```python
from build123d import *

# Parameters (mm, degrees)
EXTRUDE_1_DEPTH      = 20
CHAMFER_1_SIZE       = 2
SKETCH_5_R           = 5
CUT_EXTRUDE_4_DEPTH  = 5
SKETCH_3_W           = 36
SKETCH_3_H           = 10
CUT_EXTRUDE_2_DEPTH  = 200.103917213
CUT_EXTRUDE_3_DEPTH  = 195.273950902
CHAMFER_2_SIZE       = 2
CHAMFER_3_SIZE       = 2
CHAMFER_4_SIZE       = 2
CUT_EXTRUDE_START    = -20
SKETCH_8_W           = 28.3
SKETCH_8_H           = 31
CUT_EXTRUDE_5_DEPTH  = 10
SKETCH_9_R           = 11.25
CUT_EXTRUDE_6_DEPTH  = 2.1
SKETCH_9_3_R         = 1.35
CUT_EXTRUDE_7_DEPTH  = 194.500304907
CUT_EXTRUDE_8_DEPTH  = 195.273950902
SKETCH_11_W          = 21.182127439
SKETCH_11_H          = 11.878785241
CUT_EXTRUDE_9_DEPTH  = 200.103917213
SKETCH_12_R          = 9
CUT_EXTRUDE_10_DEPTH = 194.62019006
SKETCH_13_R          = 7.05
CUT_EXTRUDE_11_DEPTH = 4.1
SKETCH_14_R          = 22.5
CUT_EXTRUDE_12_DEPTH = 1


with BuildPart() as part:
    # 草图1 → 凸台-拉伸1 (new body)
    with BuildSketch(Plane.XY):
        with BuildLine():
            Line((0, 15), (170, 15))
            ThreePointArc((170, 15), (185, 0), (170, -15))
            Line((170, -15), (61.353463239, -15))
            ThreePointArc((61.353463239, -15), (56.922725161, -17.682984659), (57.247028001, -22.852575965))
            ThreePointArc((57.247028001, -22.852575965), (40, -55.833395016), (22.752971999, -22.852575965))
            ThreePointArc((22.752971999, -22.852575965), (23.077274839, -17.682984659), (18.646536761, -15))
            Line((18.646536761, -15), (0, -15))
            Line((0, -15), (0, 15))
        make_face()
    extrude(amount=EXTRUDE_1_DEPTH)

    # 倒角1
    chamfer_1_edges = [part.edges().sort_by_distance(p)[0] for p in [
        (0, -15, 10),
        (0, 15, 10),
    ]]
    chamfer(chamfer_1_edges, length=CHAMFER_1_SIZE)

    # 草图5 → 切除-拉伸4 (cut)
    with BuildSketch(Plane(origin=(0, 0, 0), x_dir=(-1, 0, 0), z_dir=(0, 0, -1))):
        with Locations((-170, 0)):
            Circle(SKETCH_5_R)
    cut_extrude_4 = extrude(amount=-CUT_EXTRUDE_4_DEPTH, mode=Mode.SUBTRACT)

    # 草图3 → 切除-拉伸2 (cut, through all)
    with BuildSketch(Plane(origin=(0, 15, 0), x_dir=(1, 0, 0), z_dir=(0, 1, 0))):
        with Locations((170, -10)):
            Rectangle(SKETCH_3_W, SKETCH_3_H)
    extrude(amount=-CUT_EXTRUDE_2_DEPTH, mode=Mode.SUBTRACT)

    # 草图4 → 切除-拉伸3 (cut, through all)
    with BuildSketch(Plane(origin=(0, 0, 0), x_dir=(-1, 0, 0), z_dir=(0, 0, -1))):
        with BuildLine():
            Line((-40, -7.5), (-137, -7.5))
            ThreePointArc((-137, -7.5), (-144.5, 0), (-137, 7.5))
            Line((-137, 7.5), (-40, 7.5))
            ThreePointArc((-40, 7.5), (-32.5, 0), (-40, -7.5))
        make_face()
    extrude(amount=-CUT_EXTRUDE_3_DEPTH, mode=Mode.SUBTRACT)

    # 倒角2
    chamfer_2_edges = [part.edges().sort_by_distance(p)[0] for p in [
        (32.5, 0, 20),
        (88.5, -7.5, 20),
        (144.5, 0, 20),
        (88.5, 7.5, 20),
        (32.5, 0, 0),
        (88.5, 7.5, 0),
        (144.5, 0, 0),
        (88.5, -7.5, 0),
    ]]
    chamfer(chamfer_2_edges, length=CHAMFER_2_SIZE)

    # 倒角3
    chamfer_3_edges = [part.edges().sort_by_distance(p)[0] for p in [
        (10.323268381, -15, 0),
        (23.077274839, -17.682984659, 0),
        (40, -55.833395016, 0),
        (56.922725161, -17.682984659, 0),
        (115.676731619, -15, 0),
        (185, 0, 0),
        (86, 15, 0),
    ]]
    chamfer(chamfer_3_edges, length=CHAMFER_3_SIZE)

    # 倒角4
    chamfer_4_edges = [part.edges().sort_by_distance(p)[0] for p in [
        (10.323268381, -15, 20),
        (23.077274839, -17.682984659, 20),
        (40, -55.833395016, 20),
        (56.922725161, -17.682984659, 20),
        (115.676731619, -15, 20),
        (185, 0, 20),
        (86, 15, 20),
    ]]
    chamfer(chamfer_4_edges, length=CHAMFER_4_SIZE)

    # 镜向1: 切除-拉伸4 across plane
    add(cut_extrude_4.mirror(Plane(origin=(0, 0, 10), x_dir=(1, 0, 0), z_dir=(0, 0, -1))), mode=Mode.SUBTRACT)

    # 草图8 → 切除-拉伸5 (cut)
    with BuildSketch(Plane(origin=(0, 0, 0), x_dir=(-1, 0, 0), z_dir=(0, 0, -1)).offset(CUT_EXTRUDE_START)):
        with Locations((-15, 0)):
            Rectangle(SKETCH_8_W, SKETCH_8_H)
    extrude(amount=CUT_EXTRUDE_5_DEPTH, mode=Mode.SUBTRACT)

    # 草图9 → 切除-拉伸6 (cut)
    with BuildSketch(Plane.XY.offset(10)):
        with Locations((15, 0)):
            Circle(SKETCH_9_R)
    extrude(amount=-CUT_EXTRUDE_6_DEPTH, mode=Mode.SUBTRACT)

    # 草图9<3> → 切除-拉伸7 (cut, through all)
    with BuildSketch(Plane.XY.offset(10)):
        with Locations((26.5, 11.5)):
            Circle(SKETCH_9_3_R)
        with Locations((3.5, 11.5)):
            Circle(SKETCH_9_3_R)
        with Locations((3.5, -11.5)):
            Circle(SKETCH_9_3_R)
        with Locations((26.5, -11.5)):
            Circle(SKETCH_9_3_R)
    extrude(amount=-CUT_EXTRUDE_7_DEPTH, mode=Mode.SUBTRACT)

    # 草图10 → 切除-拉伸8 (cut, through all)
    with BuildSketch(Plane.XY.offset(20)):
        with BuildLine():
            Line((42.664582519, -31.783395016), (37.335417481, -31.783395016))
            ThreePointArc((37.335417481, -31.783395016), (38.32504615, -38.520810046), (44.05, -34.833395016))
            ThreePointArc((44.05, -34.833395016), (43.68741503, -33.158441166), (42.664582519, -31.783395016))
        make_face()
    extrude(amount=-CUT_EXTRUDE_8_DEPTH, mode=Mode.SUBTRACT)

    # 草图11 → 切除-拉伸9 (cut, through all)
    with BuildSketch(Plane(origin=(0, 15, 0), x_dir=(1, 0, 0), z_dir=(0, 1, 0))):
        with Locations((1.235913402, -15.939392621)):
            Rectangle(SKETCH_11_W, SKETCH_11_H)
    extrude(amount=-CUT_EXTRUDE_9_DEPTH, mode=Mode.SUBTRACT)

    # 草图12 → 切除-拉伸10 (cut, through all)
    with BuildSketch(Plane.XY.offset(7.9)):
        with Locations((15, 0)):
            Circle(SKETCH_12_R)
    extrude(amount=-CUT_EXTRUDE_10_DEPTH, mode=Mode.SUBTRACT)

    # 草图13 → 切除-拉伸11 (cut)
    with BuildSketch(Plane(origin=(0, 0, 15), x_dir=(-1, 0, 0), z_dir=(0, 0, -1))):
        with Locations((-170, 0)):
            Circle(SKETCH_13_R)
    cut_extrude_11 = extrude(amount=-CUT_EXTRUDE_11_DEPTH, mode=Mode.SUBTRACT)

    # 镜向2: 切除-拉伸11 across plane
    add(cut_extrude_11.mirror(Plane(origin=(0, 0, 10), x_dir=(1, 0, 0), z_dir=(0, 0, -1))), mode=Mode.SUBTRACT)

    # 草图14 → 切除-拉伸12 (cut)
    with BuildSketch(Plane.XY.offset(20)):
        with Locations((40, -34.833395016)):
            Circle(SKETCH_14_R)
    cut_extrude_12 = extrude(amount=-CUT_EXTRUDE_12_DEPTH, mode=Mode.SUBTRACT)

    # 镜向3: 切除-拉伸12 across plane
    add(cut_extrude_12.mirror(Plane(origin=(0, 0, 10), x_dir=(1, 0, 0), z_dir=(0, 0, -1))), mode=Mode.SUBTRACT)


solid = part.part
```
Geometry: final body of the model. Coordinates: model frame, mm. A direction names the side the tool comes from. Give positions to 0.01 mm unless a question says otherwise; leave off trailing zeros. Loops run counter-clockwise (first coordinate to the right, second up) from the corner with the lowest first, then second, coordinate; pieces in that order, holes last. Notation, with made-up numbers: (22, -20) -> (47, -20) arc R29 ccw to (47, 14) -> close; hole circle Ø5 at (71.5, -27). An arc over 180 degrees is marked (long way). Use CSV: the item, a comma, the result in double quotes.
(1) First-contact query: P1, Ø20, axis at x = 49.5, y = -33.5, coming from the +Z side; P2, Ø8, axis at x = 113.5, z = 9, coming from the -Y side; P3, Ø5, axis at x = 40, y = -34.83, coming from the -Z side; P4, Ø1, axis at x = 27.5, z = 4, coming from the -Y side. Flat tips, straight axial feed; report the tip coordinate or a pass-through.
From the geometry:
P1,"z = 19"
P2,"y = -15"
P3,"through"
P4,"y = -52.07"
(2) Cut plane B-B (x = 129.5). Output: boundary loops of the cut face in (y, z), plus the area to 3 significant figures.
From the geometry:
outline,"(-15, 2) -> (-13, 0) -> (-9.5, 0) -> (-7.5, 2) -> (-7.5, 18) -> (-9.5, 20) -> (-13, 20) -> (-15, 18) -> close; (7.5, 2) -> (9.5, 0) -> (13, 0) -> (15, 2) -> (15, 18) -> (13, 20) -> (9.5, 20) -> (7.5, 18) -> close"
area,"284 mm^2"
(3) Access query for faces 1 (the face through (144.8, -0.2, 1.7)), 2 (the face through (163.276, 2.118, 17.021)), 3 (the face through (10, -15, 6)), 4 (the face through (25, -15.5, 15)), 5 (the face through (88, -7.5, 10)). Directions: +Z, -Z, +X, -X, +Y, -Y. A direction counts if a zero-diameter tool reaches every point of the face in a straight line with its end or side. Return the directions, or none.
From the geometry:
face 1,"-Z"
face 2,"none"
face 3,"+Z, -Z, -X, -Y"
face 4,"+Z, -X, +Y"
face 5,"+Z, -Z"
(4) Pull-direction query (Z, two-part tool) for faces 6 (the face through (172, 5, 19.1)), 7 (the face through (172, 5, 0.9)), 8 (the face through (56.959, -17.616, 9.888)), 9 (the face through (5, 7, 10)); classes: released by +Z, released by -Z, zero draft, split by the parting line, or undercut.
From the geometry:
face 6,"undercut"
face 7,"undercut"
face 8,"zero draft"
face 9,"released by +Z"
(5) Ray query, line 1 along Y through (x, z) = (3.5, 6.5); line 2 along X through (y, z) = (0, 19.3); line 3 along Y through (x, z) = (139.5, 10). Return the intervals inside material, ascending. Write a range as [from, to].
From the geometry:
line 1,"[-15, -12.85], [-10.15, 10.15], [12.85, 15]"
line 2,"[29.15, 31.2], [145.8, 165], [175, 183.7]"
line 3,"[-15, -7.07], [7.07, 15]"
(6) Cut plane A-A (x = 15). Output: boundary loops of the cut face in (y, z), plus the area to 3 significant figures.
From the geometry:
outline,"(-15, 2) -> (-13, 0) -> (-9, 0) -> (-9, 7.9) -> (-11.25, 7.9) -> (-11.25, 10) -> (-15, 10) -> close; (9, 0) -> (13, 0) -> (15, 2) -> (15, 10) -> (11.25, 10) -> (11.25, 7.9) -> (9, 7.9) -> close"
area,"107 mm^2"
